from build123d import *

# Parameters (mm, degrees)
CROQUIS1_R              = 23.9
CROQUIS1_R_2            = 8.1
SALIENTE_EXTRUIR1_DEPTH = 5
CROQUIS1_3_R            = 30
CROQUIS1_3_R_2          = 23.9
CROQUIS1_3_R_3          = 8.1
SALIENTE_EXTRUIR2_DEPTH = 5
CROQUIS1_4_R            = 30
CROQUIS1_4_R_2          = 23.9
SALIENTE_EXTRUIR3_DEPTH = 15


with BuildPart() as part:
    # Croquis1 → Saliente-Extruir1 (new body)
    with BuildSketch(Plane(origin=(0, 0, 0), x_dir=(1, 0, 0), z_dir=(0, 1, 0))):
        Circle(CROQUIS1_R)
        Circle(CROQUIS1_R_2, mode=Mode.SUBTRACT)
    extrude(amount=SALIENTE_EXTRUIR1_DEPTH)

    # Croquis1_3 → Saliente-Extruir2 (add)
    with BuildSketch(Plane(origin=(0, 0, 0), x_dir=(1, 0, 0), z_dir=(0, 1, 0))):
        Circle(CROQUIS1_3_R)
        Circle(CROQUIS1_3_R_2, mode=Mode.SUBTRACT)
        Circle(CROQUIS1_3_R_2)
        Circle(CROQUIS1_3_R_3, mode=Mode.SUBTRACT)
    extrude(amount=-SALIENTE_EXTRUIR2_DEPTH)

    # Croquis1_4 → Saliente-Extruir3 (add)
    with BuildSketch(Plane(origin=(0, 0, 0), x_dir=(1, 0, 0), z_dir=(0, 1, 0))):
        Circle(CROQUIS1_4_R)
        Circle(CROQUIS1_4_R_2, mode=Mode.SUBTRACT)
    extrude(amount=-SALIENTE_EXTRUIR3_DEPTH)


solid = part.part
Here's how the part is built. I have some questions about the finished solid (model axes, mm). A direction names the side the tool comes from. Give positions to 0.01 mm unless a question says otherwise; leave off trailing zeros. Order: outer loops, then holes, each group sorted by start corner. A loop starts at its lowest first (then second) coordinate and runs counter-clockwise, first axis right, second up. Notation, with made-up numbers: M 39.25,31.25 L 88.25,31.25 A28 ccw 88.25,58.25 Z; hole C -1.75,-38 d5. An arc over 180 degrees is marked long. Answer as a JSON object with one key per item and string values. Group by question number.
1) We'd pull the mould along Z, two halves only. Please class faces 4 (the cylindrical face through (-29.97, -7.4, -1.32)), 5 (the flat face through (10, -5, 0)), 6 (the flat face through (0, 5, 10)): pulls with the +Z half, pulls with the -Z half, needs draft (parallel to the pull), parting line crosses it, or undercut.
2) Please list where these lines run through material, in increasing order: L1, parallel to X at y = -2, z = 0; L2, parallel to Z at x = 0, y = -10.5; L3, parallel to Z at x = -15, y = -12. Write a range as [from, to].
3) I'm going to push flat-ended pins straight in: pin 1 Ø5 at (x, y) = (-10.5, 0.5) entering from +Z; pin 2 Ø1 at (y, z) = (-8, -4.5) entering from +X; pin 3 Ø1.5 at (x, y) = (22, -9.5) entering from -Z; pin 4 Ø8 at (x, z) = (-22, 12.5) entering from +Y. Where does each tip first touch, or does it pass through?
4) Suppose I cut it at D-D, the plane z = 10.5. Write out the boundary of the cut face in (x, y).
5) Suppose I cut it at B-B, the plane z = 0. Write out the boundary of the cut face in (x, y), plus the area to 3 significant figures.
6) Suppose I cut it at C-C, the plane y = 1. Write out the boundary of the cut face in (x, z), plus the area to 3 significant figures.
7) Suppose I cut it at A-A, the plane x = 0. Write out the boundary of the cut face in (y, z), plus the area to 3 significant figures.
8) On a 3-axis mill with a long thin cutter (end or side, diameter ignored), from which of +Z, -Z, +X, -X, +Y, -Y can I reach the whole of each face in a straight line? I mean faces 1 (the flat face through (-20.14, -15, 13.19)), 2 (the cylindrical face through (12.85, 2.46, -20.15)), 3 (the cylindrical face through (12.85, -9.93, -20.15)). Say none if no direction works.
Results found:
{
 "1": {"face 4": "parting line crosses it", "face 5": "undercut", "face 6": "needs draft"},
 "2": {"L1": "[-30, -8.1], [8.1, 30]", "L2": "[-30, -23.9], [23.9, 30]", "L3": "[-25.98, -18.61], [18.61, 25.98]"},
 "3": {"pin 1": "z = 28.9", "pin 2": "x = 29.73", "pin 3": "z = -21.18", "pin 4": "y = 5"},
 "4": {"outline": "M -28.1,-15 L -21.47,-15 L -21.47,-5 L 21.47,-5 L 21.47,-15 L 28.1,-15 L 28.1,0 L 21.47,0 L 21.47,5 L -21.47,5 L -21.47,0 L -28.1,0 Z"},
 "5": {"outline": "M -30,-15 L -23.9,-15 L -23.9,-5 L -8.1,-5 L -8.1,5 L -23.9,5 L -23.9,0 L -30,0 Z; M 8.1,-5 L 23.9,-5 L 23.9,-15 L 30,-15 L 30,0 L 23.9,0 L 23.9,5 L 8.1,5 Z", "area": "499 mm²"},
 "6": {"outline": "C 0,0 d47.8; hole C 0,0 d16.2", "area": "1,590 mm²"},
 "7": {"outline": "M -15,-30 L 0,-30 L 0,-23.9 L 5,-23.9 L 5,-8.1 L -5,-8.1 L -5,-23.9 L -15,-23.9 Z; M -15,23.9 L -5,23.9 L -5,8.1 L 5,8.1 L 5,23.9 L 0,23.9 L 0,30 L -15,30 Z", "area": "499 mm²"},
 "8": {"face 1": "+Z, -Z, +X, -X, -Y", "face 2": "+Y", "face 3": "-Y"}
}
